Autodesk Inventor part; units mm, degrees
ref_plane "YZ Plane" through (0, 0, 0) normal (1, 0, 0) x (0, 1, 0)
ref_plane "XZ Plane" through (0, 0, 0) normal (0, 1, 0) x (-1, 0, 0)
ref_plane "XY Plane" through (0, 0, 0) normal (0, 0, 1) x (1, 0, 0)
sketch "Sketch1" plane through (0, 0, 0) normal (0, 0, 1) x (1, 0, 0)
  line L0 (0, 0) -> (23, 0)
  line L1 (23, 0) -> (23, 43.5)
  line L2 (23, 43.5) -> (0, 43.5)
  line L3 (0, 43.5) -> (0, 0)
  dimension "d0" = 23
  dimension "d1" = 43.5
extrude "Extrusion1" add sketch "Sketch1" along normal blind 3
sketch "Sketch6" plane through (0, 0, 0) normal (0, 0, -1) x (-1, 0, 0)
  line L0 (0, 0) -> (-2.5, 0)
  line L1 (-2.5, 0) -> (-2.5, 32.5)
  line L2 (-2.5, 32.5) -> (0, 32.5)
  line L3 (0, 32.5) -> (0, 0)
  dimension "d17" = 2.5
  dimension "d18" = 32.5
extrude "Extrusion5" add sketch "Sketch6" along normal blind 23.5
sketch "Sketch7" plane through (2.5, 0, 0) normal (1, 0, 0) x (0, 0, -1)
  line L0 (23.5, 0) -> (23.5, 32.5)
  line L1 (0, 32.5) -> (23.5, 32.5)
  line L2 (23.5, 0) -> (21.5, 0)
  line L3 (21.5, 0) -> (21.5, 32.5)
  line L4 (21.5, 32.5) -> (23.5, 32.5)
  line L5 (23.5, 32.5) -> (23.5, 0)
  point P0 (0, 0)
  dimension "d21" = 2
extrude "Extrusion6" add sketch "Sketch7" along normal blind 20.5
sketch "Sketch8" plane through (0, 0, 3) normal (0, -1, 0) x (1, 0, 0)
  line L0 (2.5, -3) -> (23, -3)
  line L1 (23, -3) -> (23, 0)
  line L2 (0, 0) -> (23, 0)
  line L3 (0, 0) -> (0, -26.5)
  line L4 (0, -26.5) -> (23, -26.5)
  line L5 (23, -24.5) -> (23, -26.5)
  line L6 (2.5, -24.5) -> (23, -24.5)
  line L7 (2.5, -3) -> (2.5, -24.5)
  line L8 (23, -3) -> (23, -10)
  line L9 (23, -10) -> (7.5, -10)
  line L10 (7.5, -10) -> (7.5, -23.5)
  line L11 (7.5, -23.5) -> (23, -23.5)
  line L12 (23, -23.5) -> (23, -24.5)
  point P0 (0, -3)
  dimension "d24" = 7
  dimension "d25" = 1
  dimension "d26" = 5
extrude "Extrusion7" add sketch "Sketch8" against normal blind 2.5 contours L0 L8 L9 L10 L11 L12 L6 L7
sketch "Sketch10" plane through (0, 2.5, 3) normal (0, 1, 0) x (1, 0, 0)
  circle A0 centre (13, 7.5) radius 2
  line L0 (23, 3) -> (23, 10)
  line L1 (23, 3) -> (0, 3)
  dimension "d35" = 10
  dimension "d36" = 4.5
  dimension "d37" = 4
extrude "Extrusion9" cut sketch "Sketch10" against normal blind 2.5
sketch "Sketch11" plane through (0, 0, 3) normal (0, 0, 1) x (1, 0, 0)
  circle A0 centre (6, 40.5) radius 1.75
  circle A1 centre (20, 40.5) radius 1.75
  line L0 (0, 43.5) -> (0, 0)
  line L1 (23, 0) -> (23, 43.5)
  line L2 (0, 0) -> (23, 0)
  dimension "d40" = 3.5
  dimension "d41" = 3.5
  dimension "d42" = 14
  dimension "d44" = 3
  dimension "d45" = 40.5
extrude "Extrusion10" cut sketch "Sketch11" against normal blind 3
sketch "Sketch12" plane through (0, 0, 3) normal (0, -1, 0) x (1, 0, 0)
  line L0 (23, -23.5) -> (7.5, -23.5)
  line L1 (7.5, -23.5) -> (3.5, -23.5)
  line L2 (3.5, -23.5) -> (3.5, -17.5)
  line L3 (3.5, -17.5) -> (7.5, -17.5)
  line L4 (7.5, -17.5) -> (7.5, -23.5)
  point P0 (0, -3)
  dimension "d48" = 4
  dimension "d49" = 6
extrude "Extrusion11" cut sketch "Sketch12" against normal blind 2.5
equation "\"d41\" = d40"
properties part number "SOPORTE_HOTEND"
Read the model definition and answer for the solid it produces. Units are mm, in the model's axes. A direction names the side the tool comes from. Round coordinates to 2 decimals unless told otherwise and drop trailing zeros. Order: outer loops, then holes, each group sorted by start corner. A loop starts at its lowest first (then second) coordinate and runs counter-clockwise, first axis right, second up.
1) For faces 1 (the face through (15, 1, -7)), 2 (the face through (2, 32.5, -16)), 3 (the face through (12, 43.5, 1)), 4 (the face through (10, 2.5, -6)), determine the directions among +Z, -Z, +X, -X, +Y, -Y from which every point of the face is accessible in a straight line to the end or side of a thin tool.
2) The part is cut by section D-D on y = 15.5. Write down the section's boundary in (x, z).
3) The part is cut by section A-A on x = 13. Write down the section's boundary in (y, z).
4) Flat-ended cylindrical pins translate along their axes: pin 1 (3 mm diameter, centred on y = 1, z = -17.5, fed in from +X); pin 2 (5 mm diameter, centred on y = 35.5, z = -11, fed in from -X); pin 3 (10 mm diameter, centred on x = 5.5, z = -15.5, fed in from +Y); pin 4 (4.5 mm diameter, centred on x = 6, y = 40.5, fed in from -Z). Find the tip coordinate at first contact, or state that the pin passes through.
5) The part is cut by section C-C on y = 40.5. Write down the section's boundary in (x, z), plus the area to 3 significant figures.
6) The part is cut by section B-B on z = -4.5. Write down the section's boundary in (x, y).
7) The mould has two halves that part along Z. Classify faces 5 (the face through (11, 16, -23.5)), 6 (the face through (0, 17, -10)), 7 (the face through (11, 23, 0)), 8 (the face through (11.4, 1.3, -3.3)): released by +Z, released by -Z, zero draft, split by the parting line, or undercut.
8) Straight lines are drawn through the part: L1, parallel to Z at x = 13, y = 1.8; L2, parallel to X at y = 1.25, z = -4.5; L3, parallel to Z at x = 9.5, y = 9. For each, find the intervals that lie inside material, in ascending order.
Resolved:
1. face 1: +X, +Y, -Y
1. face 2: -Z, +X, -X, +Y
1. face 3: +Z, -Z, +X, -X, +Y
1. face 4: +X, +Y
2. outline: (0, -23.5) - (23, -23.5) - (23, -21.5) - (2.5, -21.5) - (2.5, 0) - (23, 0) - (23, 3) - (0, 3) - close
3. outline: (0, -23.5) - (32.5, -23.5) - (32.5, -21.5) - (2.5, -21.5) - (2.5, -20.5) - (0, -20.5) - close; (0, -7) - (2.5, -7) - (2.5, -6.5) - (0, -6.5) - close; (0, -2.5) - (2.5, -2.5) - (2.5, 0) - (43.5, 0) - (43.5, 3) - (0, 3) - close
4. pin 1: stops at x = 3.5
4. pin 2: passes through
4. pin 3: stops at y = 32.5
4. pin 4: stops at z = 0
5. outline: (0, 0) - (4.25, 0) - (4.25, 3) - (0, 3) - close; (7.75, 0) - (18.25, 0) - (18.25, 3) - (7.75, 3) - close; (21.75, 0) - (23, 0) - (23, 3) - (21.75, 3) - close
5. area: 48.0 mm2
6. outline: (0, 0) - (11, 0) - (11, 2.5) - (2.5, 2.5) - (2.5, 32.5) - (0, 32.5) - close; (15, 0) - (23, 0) - (23, 2.5) - (15, 2.5) - close
7. face 5: released by -Z
7. face 6: zero draft
7. face 7: undercut
7. face 8: undercut
8. L1: z = -23.5 to -20.5, -7 to -6.5, -2.5 to 3
8. L2: x = 0 to 11, 15 to 23
8. L3: z = -23.5 to -21.5, 0 to 3
